Autodesk Inventor part; units mm, degrees
ref_plane "YZ Plane" through (0, 0, 0) normal (1, 0, 0) x (0, 1, 0)
ref_plane "XZ Plane" through (0, 0, 0) normal (0, 1, 0) x (-1, 0, 0)
ref_plane "XY Plane" through (0, 0, 0) normal (0, 0, 1) x (1, 0, 0)
sketch "스케치1" plane through (0, 0, 0) normal (0, 1, 0) x (-1, 0, 0)
  line L0 (18, -14) -> (-20, -14)
  line L1 (-20, -14) -> (-20, 14)
  line L2 (-20, 14) -> (18, 14)
  line L3 (18, 14) -> (18, -14)
  point P0 (0, 0)
  dimension "d0" = 28
  dimension "d1" = 14
  dimension "d2" = 38
  dimension "d3" = 18
extrude "돌출1" add sketch "스케치1" along normal blind 50
sketch "스케치2" plane through (0, 50, 0) normal (0, 1, 0) x (1, 0, 0)
  line L0 (20, 14) -> (-18, 14)
  line L1 (-18, -14) -> (20, -14)
  line L2 (-18, 14) -> (-13.01, 14)
  line L3 (-13.01, 14) -> (-13.01, -14)
  line L4 (-13.01, -14) -> (-18, -14)
  line L5 (-18, -14) -> (-18, 14)
  line L6 (20, -14) -> (15.01, -14)
  line L7 (15.01, -14) -> (15.01, 14)
  line L8 (15.01, 14) -> (20, 14)
  line L9 (20, 14) -> (20, -14)
  point P0 (0, 0)
  dimension "d6" = 4.99
  dimension "d7" = 4.99
extrude "돌출2" add sketch "스케치2" along normal blind 5 contours L9 L1 L7 L0 | L3 L1 L5 L0
sketch "스케치4" plane through (20, 0, 14) normal (1, 0, 0) x (0, 0, -1)
  circle A0 centre (3, 52) radius 1.5
  circle A1 centre (25, 52) radius 1.5
  line L0 (0, 55) -> (28, 55)
  line L1 (28, 0) -> (28, 55)
  line L2 (0, 0) -> (0, 55)
  point P0 (14, 0)
  dimension "d24" = 3
  dimension "d25" = 3
  dimension "d26" = 3
  dimension "d27" = 3
  dimension "d28" = 3
  dimension "d29" = 3
extrude "돌출4" cut sketch "스케치4" against normal blind 80
sketch "스케치5" plane through (0, 0, 0) normal (0, -1, 0) x (1, 0, 0)
  line L0 (20, -14) -> (20, 14)
  line L1 (-18, -14) -> (20, -14)
  line L2 (20, 14) -> (15.01, 14)
  line L3 (15.01, 14) -> (15.01, -14)
  line L4 (15.01, -14) -> (20, -14)
  line L5 (20, -14) -> (20, 14)
  line L6 (-18, 14) -> (-13.01, 14)
  line L7 (-13.01, 14) -> (-13.01, -14)
  line L8 (-13.01, -14) -> (-18, -14)
  line L9 (-18, -14) -> (-18, 14)
  point P0 (0, 0)
  dimension "d32" = 4.99
  dimension "d33" = 4.99
extrude "돌출5" add sketch "스케치5" along normal blind 5
sketch "스케치6" plane through (20, 55, 14) normal (1, 0, 0) x (0, 0, -1)
  circle A0 centre (25, -57) radius 1.5
  circle A1 centre (3, -57) radius 1.5
  line L0 (28, -60) -> (0, -60)
  line L1 (28, 0) -> (28, -60)
  line L2 (0, 0) -> (0, -60)
  point P0 (14, -55)
  dimension "d36" = 3
  dimension "d37" = 3
  dimension "d38" = 3
  dimension "d39" = 3
  dimension "d40" = 3
  dimension "d41" = 3
extrude "돌출6" cut sketch "스케치6" against normal blind 80
properties part number "upperarm"
Geometry: final body of the model. Coordinates: model frame, mm. A direction names the side the tool comes from. Round coordinates to 2 decimals unless told otherwise and drop trailing zeros. Order: outer loops, then holes, each group sorted by start corner. A loop starts at its lowest first (then second) coordinate and runs counter-clockwise, first axis right, second up. Notation, with made-up numbers: (80.5, 76) -> (103.5, 76) arc R19 ccw to (103.5, 100) -> close; hole circle Ø3 at (-38.75, 18). An arc over 180 degrees is marked (long way). Use one line per item in the form item = value.
(1) Section B-B on z = 11. Return loops of the section in (x, y).
Results list:
outline = (-18, -5) -> (-13.01, -5) -> (-13.01, -3.5) -> (-18, -3.5) -> close; (-18, -0.5) -> (-13.01, -0.5) -> (-13.01, 0) -> (15.01, 0) -> (15.01, -0.5) -> (20, -0.5) -> (20, 50.5) -> (15.01, 50.5) -> (15.01, 50) -> (-13.01, 50) -> (-13.01, 50.5) -> (-18, 50.5) -> close; (-18, 53.5) -> (-13.01, 53.5) -> (-13.01, 55) -> (-18, 55) -> close; (15.01, -5) -> (20, -5) -> (20, -3.5) -> (15.01, -3.5) -> close; (15.01, 53.5) -> (20, 53.5) -> (20, 55) -> (15.01, 55) -> close
(2) Access query for faces 4 (the face through (1, 50, 0)), 5 (the face through (1, 25, 14)), 6 (the face through (-13.01, -2, 0)). Directions: +Z, -Z, +X, -X, +Y, -Y. A direction counts if a zero-diameter tool reaches every point of the face in a straight line with its end or side. Return the directions, or none.
Results list:
face_4 = +Z, -Z, +Y
face_5 = +Z, +X, -X, +Y, -Y
face_6 = +Z, -Z, -Y
(3) Ray query, probe 1 along Y at (x, z) = (17.75, 11); probe 2 along X at (y, z) = (51.5, -5); probe 3 along Y at (x, z) = (0, 1). Return the intervals inside material, ascending. Write a range as [from, to].
Results list:
probe_1 = [-5, -3.5], [-0.5, 50.5], [53.5, 55]
probe_2 = [-18, -13.01], [15.01, 20]
probe_3 = [0, 50]
(4) First-contact query: pin 1 Ø2.5 at (y, z) = (52, 11) entering from +X; pin 2 Ø8 at (x, z) = (-0.5, 5) entering from +Y; pin 3 Ø14 at (x, z) = (6, 4) entering from -Y. Flat tips, straight axial feed; report the tip coordinate or a pass-through.
Results list:
pin_1 = through
pin_2 = 50
pin_3 = 0
(5) Section D-D on x = 4. Return loops of the section in (y, z).
Results list:
outline = (0, -14) -> (50, -14) -> (50, 14) -> (0, 14) -> close
(6) Section C-C on z = -6. Return loops of the section in (x, y), and give its area (3 significant figures).
Results list:
outline = (-18, -5) -> (-13.01, -5) -> (-13.01, 0) -> (15.01, 0) -> (15.01, -5) -> (20, -5) -> (20, 55) -> (15.01, 55) -> (15.01, 50) -> (-13.01, 50) -> (-13.01, 55) -> (-18, 55) -> close
area = 2,000 mm^2
(7) Section A-A on y = -2. Return loops of the section in (x, z).
Results list:
outline = (-18, -14) -> (-13.01, -14) -> (-13.01, -12.5) -> (-18, -12.5) -> close; (-18, -9.5) -> (-13.01, -9.5) -> (-13.01, 9.5) -> (-18, 9.5) -> close; (-18, 12.5) -> (-13.01, 12.5) -> (-13.01, 14) -> (-18, 14) -> close; (15.01, -14) -> (20, -14) -> (20, -12.5) -> (15.01, -12.5) -> close; (15.01, -9.5) -> (20, -9.5) -> (20, 9.5) -> (15.01, 9.5) -> close; (15.01, 12.5) -> (20, 12.5) -> (20, 14) -> (15.01, 14) -> close
(8) Draft query along Z for faces 1 (the face through (-15.47, -1.93, 12.5)), 2 (the face through (15.01, -2, 0)), 3 (the face through (1, 25, -14)). Return one class per face: pulls with the +Z half, pulls with the -Z half, needs draft (parallel to the pull), parting line crosses it, or undercut.
Results list:
face_1 = undercut
face_2 = needs draft
face_3 = pulls with the -Z half
